Part print with two shaded views. Sizes in mm from the minimum x, y, z corner. A direction names the side the tool comes from. Round coordinates to 2 decimals unless told otherwise and drop trailing zeros. Write each loop counter-clockwise with the first axis right and the second up, starting at its lowest first coordinate (ties: lowest second). Pieces come first, ordered by that corner, then holes. Notation, with made-up numbers: (78.5, 12.25) -> (92.5, 12.25) arc R21 ccw to (92.5, 41.25) -> close; hole circle Ø3 at (37.25, 82.25). An arc over 180 degrees is marked (long way). Return JSON: item names as keys, results as strings. Group by question number.
(1) Saw through at D-D (x = 25). List the corners of the cut face in (y, z), plus the area to 3 significant figures.
(2) Drill centre lines: L1, parallel to Z at x = 24.5, y = 5.08; L2, parallel to X at y = 8.5, z = 26; L3, parallel to X at y = 27, z = 19.5. Where is each one in solid material? Low to high. Write a range as from..to.
(3) Saw through at C-C (y = 5.08). List the corners of the cut face in (x, z).
(4) Saw through at B-B (z = 16). List the corners of the cut face in (x, y).
(5) Tool access for the marked faces 5 and 6: list every direction of +Z, -Z, +X, -X, +Y, -Y with a clear straight run to the whole face (end or side of a thin tool).
(6) Drop flat-ended pins along their axis: pin 1 Ø5 at (y, z) = (5.08, 7.62) entering from +X; pin 2 Ø3.5 at (x, y) = (3.81, 26.88) entering from -Z. Give the stop position or say it passes through.
(7) Saw through at A-A (z = 7.62). List the corners of the cut face in (x, y).
(8) Mould opens along X. For the marked faces 1, 2, 3 and 4 say: +X half, -X half, draft (parallel to the pull), parting line (faces both ways), or undercut.
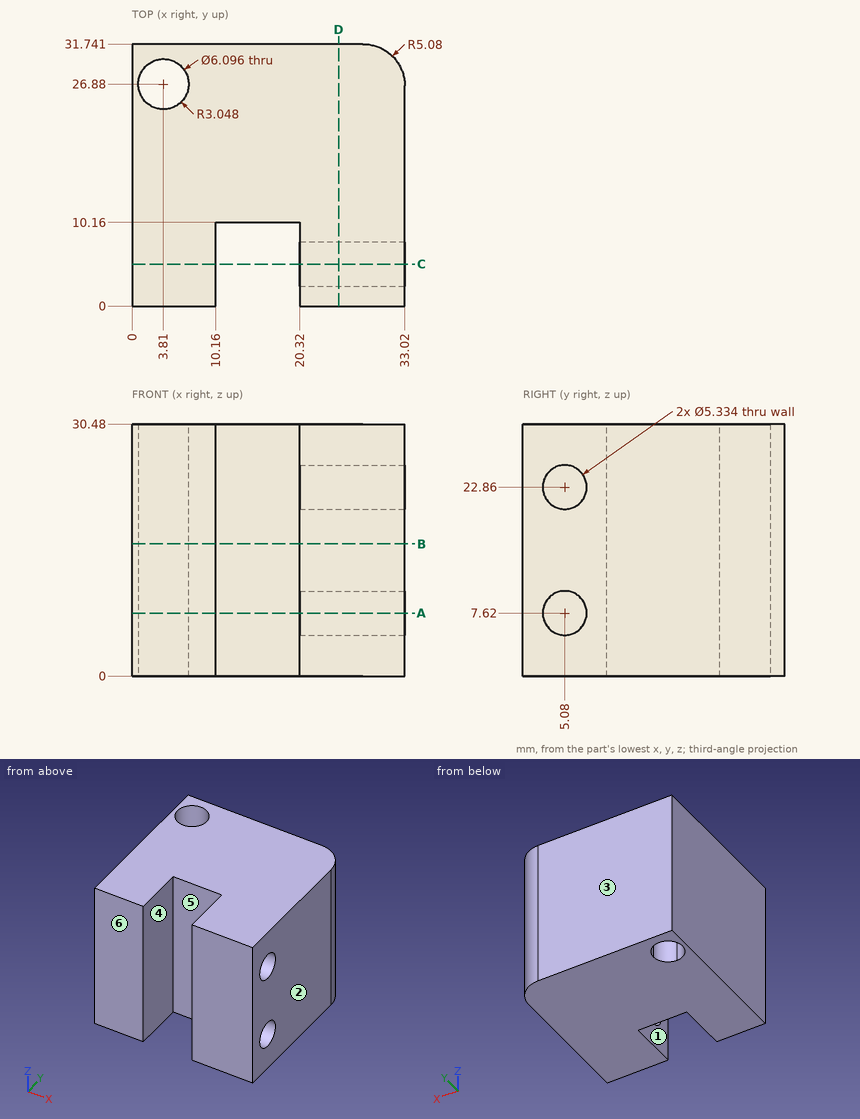
Computed values:
{
 "1": {"outline": "(0, 0) -> (31.74, 0) -> (31.74, 30.48) -> (0, 30.48) -> close; hole circle Ø5.33 at (5.08, 7.62); hole circle Ø5.33 at (5.08, 22.86)", "area": "923 mm2"},
 "2": {"L1": "0..4.95, 10.29..20.19, 25.53..30.48", "L2": "0..10.16, 20.32..33.02", "L3": "0..0.76, 6.86..33.01"},
 "3": {"outline": "(0, 0) -> (10.16, 0) -> (10.16, 30.48) -> (0, 30.48) -> close; (20.32, 0) -> (33.02, 0) -> (33.02, 4.95) -> (20.32, 4.95) -> close; (20.32, 10.29) -> (33.02, 10.29) -> (33.02, 20.19) -> (20.32, 20.19) -> close; (20.32, 25.53) -> (33.02, 25.53) -> (33.02, 30.48) -> (20.32, 30.48) -> close"},
 "4": {"outline": "(0, 0) -> (10.16, 0) -> (10.16, 10.16) -> (20.32, 10.16) -> (20.32, 0) -> (33.02, 0) -> (33.02, 26.66) arc R5.08 ccw to (27.94, 31.74) -> (0, 31.74) -> close; hole (3.81, 23.83) arc R3.05 ccw to (6.86, 26.88) arc R3.05 ccw (long way) to start"},
 "5": {"face 5": "+Z, -Z, -Y", "face 6": "+Z, -Z, +X, -X, -Y"},
 "6": {"pin 1": "x = 10.16", "pin 2": "through"},
 "7": {"outline": "(0, 0) -> (10.16, 0) -> (10.16, 10.16) -> (20.32, 10.16) -> (20.32, 7.75) -> (33.02, 7.75) -> (33.02, 26.66) arc R5.08 ccw to (27.94, 31.74) -> (0, 31.74) -> close; (20.32, 0) -> (33.02, 0) -> (33.02, 2.41) -> (20.32, 2.41) -> close; hole (3.81, 23.83) arc R3.05 ccw to (6.86, 26.88) arc R3.05 ccw (long way) to start"},
 "8": {"face 1": "undercut", "face 2": "+X half", "face 3": "draft", "face 4": "undercut"}
}
